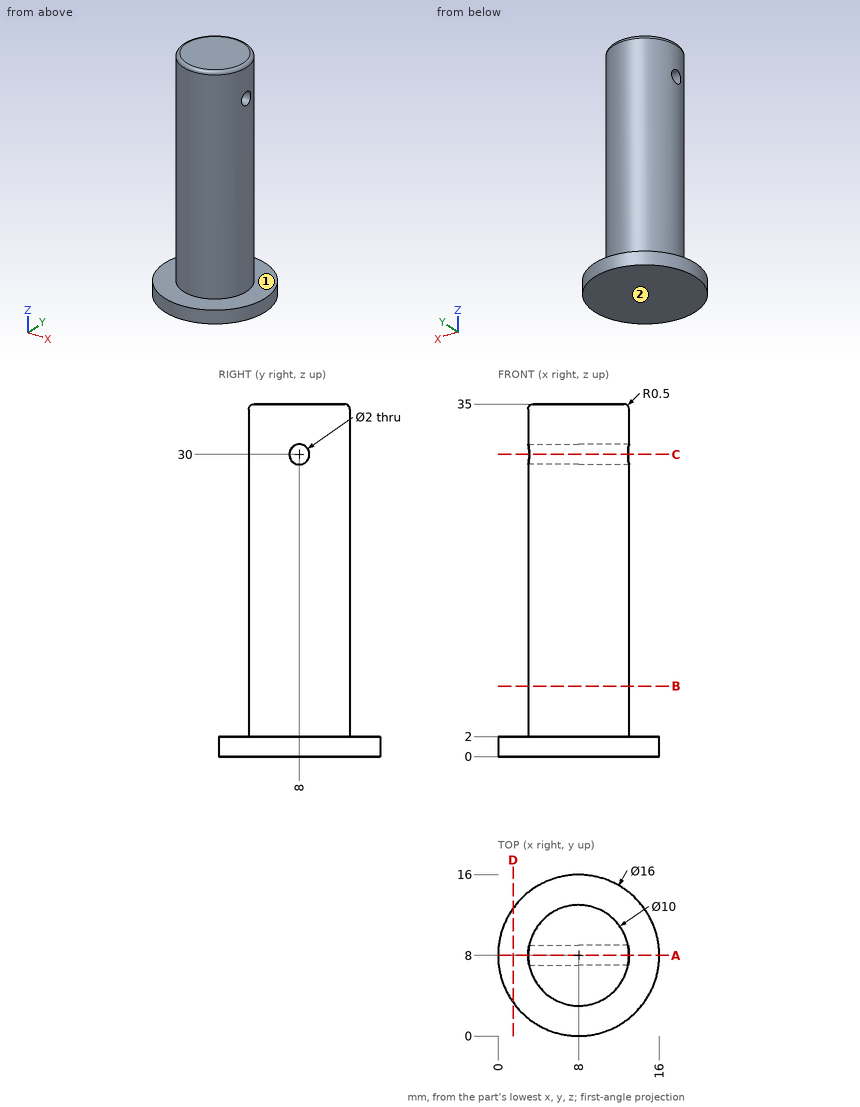
Geometry: see drawing. Coordinates: mm, zero at the bounding-box minimum. A direction names the side the tool comes from. Give positions to 0.01 mm unless a question says otherwise; leave off trailing zeros. Write each loop counter-clockwise with the first axis right and the second up, starting at its lowest first coordinate (ties: lowest second). Pieces come first, ordered by that corner, then holes. Notation, with made-up numbers: (-16, 24) - (14, 24) arc R15 cw to (14, 51) - close; hole circle Ø4 at (2.25, 88.25). An arc over 180 degrees is marked (long way). Return JSON: item names as keys, results as strings. Group by question number.
1) Section B-B on z = 7. Return the cut outline in (x, y).
2) Set-up query: the marked faces 1 and 2. Return all of +Z, -Z, +X, -X, +Y, -Y with unobstructed straight access to the full face (end or side cutting, diameter ignored); none if empty.
3) Section C-C on z = 30. Return the cut outline in (x, y).
4) Section A-A on y = 8. Return the cut outline in (x, z), plus the area to 3 significant figures.
5) Line query: line 1 (Z direction, x = 9.4, y = 8); line 2 (X direction, y = 8.25, z = 9); line 3 (Y direction, x = 5, z = 29.5). Output: solid intervals per line, ascending.
6) First-contact query: P1, Ø3, axis at y = 8, z = 30, coming from the -X side; P2, Ø8, axis at x = 8.5, y = 3.5, coming from the -Z side; P3, Ø2, axis at y = 12, z = 19, coming from the -X side; P4, Ø3, axis at x = 7, z = 18, coming from the +Y side. Flat tips, straight axial feed; report the tip coordinate or a pass-through.
7) Section D-D on x = 1.5. Return the cut outline in (y, z).
Filled in:
{
 "1": {"outline": "circle Ø10 at (8, 8)"},
 "2": {"face 1": "+Z", "face 2": "-Z, +X, -X, +Y, -Y"},
 "3": {"outline": "(3.1, 7) arc R5 ccw to (12.9, 7) - close; (3.1, 9) - (12.9, 9) arc R5 ccw to start"},
 "4": {"outline": "(0, 0) - (16, 0) - (16, 2) - (13, 2) - (13, 29) - (3, 29) - (3, 2) - (0, 2) - close; (3, 31) - (13, 31) - (13, 34.5) arc R0.5 ccw to (12.5, 35) - (3.5, 35) arc R0.5 ccw to (3, 34.5) - close", "area": "342 mm^2"},
 "5": {"line 1": "z = 0 to 29, 31 to 35", "line 2": "x = 3.01 to 12.99", "line 3": "y = 4 to 7.13, 8.87 to 12"},
 "6": {"P1": "stops at x = 3", "P2": "stops at z = 0", "P3": "stops at x = 4", "P4": "stops at y = 13"},
 "7": {"outline": "(3.34, 0) - (12.66, 0) - (12.66, 2) - (3.34, 2) - close"}
}
